from build123d import *

# Parameters (mm, degrees)
BOX005_W                  = 34.5
BOX005_H                  = 6
BOX005_DEPTH              = 9
BOX004_W                  = 85
BOX004_H                  = 55
BOX004_DEPTH              = 6.5
FUSION001_PLACEMENT_ANGLE = 25


with BuildPart() as cube010:
    # Box005 → Box005 (new body)
    with BuildSketch(Plane(origin=(7, 48, 0), x_dir=(1, 0, 0), z_dir=(0, 0, 1))):
        with Locations((17.25, 3)):
            Rectangle(BOX005_W, BOX005_H)
    extrude(amount=BOX005_DEPTH)


with BuildPart() as touchscreen:
    # Box004 → Box004 (new body)
    with BuildSketch(Plane.XY.offset(9)):
        with Locations((42.5, 27.5)):
            Rectangle(BOX004_W, BOX004_H)
    extrude(amount=BOX004_DEPTH)

    # Fusion001: union Cube010
    add(cube010.part)


with BuildPart() as touchscreen_1:
    # Fusion001 placement: moved
    add(touchscreen.part.moved(Location((12.6, 36, 56.64))).rotate(Axis((12.6, 36, 56.64), (1, 0, 0)), FUSION001_PLACEMENT_ANGLE))


solid = touchscreen_1.part
Design review of the part built by this model. Coordinates are the model's own, in mm. A direction names the side the tool comes from. Round coordinates to 2 decimals unless told otherwise and drop trailing zeros. Write each loop counter-clockwise with the first axis right and the second up, starting at its lowest first coordinate (ties: lowest second). Pieces come first, ordered by that corner, then holes. Notation, with made-up numbers: (70.25, -7.5) - (104.25, -7.5) arc R25 cw to (104.25, 7.5) - close; hole circle Ø2 at (-25, 13). An arc over 180 degrees is marked (long way). Use a Markdown table: item, result. Add a question column.
1. Clearance check with flat-ended pins moving along their axes: pin 1 (8 mm diameter, centred on y = 67, z = 79.5, fed in from +X); pin 2 (3 mm diameter, centred on y = 82, z = 83.5, fed in from +X); pin 3 (1.5 mm diameter, centred on x = 77.5, y = 66.5, fed in from +Z); pin 4 (5 mm diameter, centred on x = 35.5, y = 54, fed in from +Z). State where each tip first meets the part, or that it passes through.
2. We need section A-A (x = 50). State the section outline as (y, z) points.
3. For faces 4 (the face through (19.6, 80, 82)), 5 (the face through (54.1, 80, 82)), 6 (the face through (54.505, 80.689, 90.945)), 7 (the face through (36.608, 83.065, 83.483)), list the 3-axis set-ups (+Z, -Z, +X, -X, +Y, -Y) from which the entire face can be reached by the end or side of a thin tool; tool diameter is ignored.
4. We need section B-B (z = 89.5). State the section outline as (x, y) points.
5. We need section C-C (y = 57.5). State the section outline as (x, z) points.
6. Wall thickness on probe 1 along Y at (x, z) = (23.5, 77); probe 2 along X at (y, z) = (80, 86.5); probe 3 along Z at (x, y) = (69.5, 59): over which ranges is each line inside the solid? List them lowest first.
7. Mouldability with a two-part tool opening along Y and no side actions: class faces 1 (the face through (12.6, 55, 79)), 2 (the face through (54.505, 30.842, 67.701)), 3 (the face through (36.608, 77.628, 80.947)) as +Y half, -Y half, draft (parallel to the pull), parting line (faces both ways), or undercut.
Output:
| question | item | result |
|---|---|---|
| 1 | pin 1 | stops at x = 97.6 |
| 1 | pin 2 | stops at x = 54.1 |
| 1 | pin 3 | stops at z = 88.31 |
| 1 | pin 4 | stops at z = 83.3 |
| 2 | outline | (29.45, 70.69) - (32.2, 64.8) - (75.7, 85.08) - (79.5, 76.93) - (84.94, 79.46) - (81.14, 87.62) - (82.04, 88.04) - (79.3, 93.93) - close |
| 3 | face 4 | -Z, -X, +Y |
| 3 | face 5 | -Z, +X, +Y |
| 3 | face 6 | +Z, +X, -X, +Y |
| 3 | face 7 | +X, -X, +Y |
| 4 | outline | (12.6, 69.79) - (97.6, 69.79) - (97.6, 81.36) - (12.6, 81.36) - close |
| 5 | outline | (12.6, 76.6) - (97.6, 76.6) - (97.6, 83.77) - (12.6, 83.77) - close |
| 6 | probe 1 | y = 42.99 to 58.37, 79.47 to 79.66 |
| 6 | probe 2 | x = 19.6 to 54.1 |
| 6 | probe 3 | z = 77.3 to 84.47 |
| 7 | face 1 | draft |
| 7 | face 2 | -Y half |
| 7 | face 3 | undercut |
